Verification items for the finished model (mm, model axes). A direction names the side the tool comes from. Round coordinates to 2 decimals unless told otherwise and drop trailing zeros. Loops run counter-clockwise (first coordinate to the right, second up) from the corner with the lowest first, then second, coordinate; pieces in that order, holes last. Notation, with made-up numbers: (0, -16.5) -> (35, -16.5) arc R19 cw to (35, 16.5) -> close; hole circle Ø7 at (-38, 54). An arc over 180 degrees is marked (long way). Use CSV: the item, a comma, the result in double quotes. Start each with the question number.
```python
from build123d import *

# Parameters (mm, degrees)
SKETCH1_R           = 42.875795621
BOSS_EXTRUDE1_DEPTH = 6
BOSS_EXTRUDE2_DEPTH = 1.5
CUT_EXTRUDE1_REACH  = 62.932
CUT_EXTRUDE2_DEPTH  = 4
CIRPATTERN1_COUNT   = 4
CUT_EXTRUDE3_REACH  = 62.802
SKETCH5_R           = 1.375


with BuildPart() as part:
    # Sketch1 → Boss-Extrude1 (new body)
    with BuildSketch(Plane(origin=(0, 0, 0), x_dir=(1, 0, 0), z_dir=(0, 1, 0))):
        with Locations(Location((0, 0, 0), (0, 0, 270))):
            Circle(SKETCH1_R)
        Polygon((-20.109572639, -34.251708263), (-34.251708263, -20.109572639), (4.639164702, 18.781300326), (18.781300326, 4.639164702), align=None, mode=Mode.SUBTRACT)
    extrude(amount=BOSS_EXTRUDE1_DEPTH)

    # Sketch1<4> → Boss-Extrude2 (add)
    with BuildSketch(Plane(origin=(0, 0, 0), x_dir=(1, 0, 0), z_dir=(0, 1, 0))):
        Polygon((18.781300326, 4.639164702), (4.639164702, 18.781300326), (-0.664136157, 13.477999467), (13.477999467, -0.664136157), align=None)
        Polygon((-14.80627178, -28.948407404), (-28.948407404, -14.80627178), (-34.251708263, -20.109572639), (-20.109572639, -34.251708263), align=None)
    extrude(amount=BOSS_EXTRUDE2_DEPTH)

    # Sketch2 → Cut-Extrude1 (cut, up to next)
    with BuildSketch(Plane(origin=(0, 6, 0), x_dir=(1, 0, 0), z_dir=(0, 1, 0)), mode=Mode.PRIVATE) as cut_extrude1_sk1:
        Polygon((-32.676453, 12.877463126), (-12.877463126, 32.676453), (-8.634822439, 28.433812313), (-28.433812313, 8.634822439), align=None)
    cut_extrude1_tool1 = extrude(cut_extrude1_sk1.sketch, amount=-CUT_EXTRUDE1_REACH, mode=Mode.PRIVATE) & part.part
    add(cut_extrude1_tool1.solids().sort_by_distance((-20.655638, 6, -20.655638))[0], mode=Mode.SUBTRACT)

    # Sketch3 → Cut-Extrude2 (cut)
    with BuildSketch(Plane.XZ):
        with BuildLine():
            Line((-39.625795621, -2.5), (-39.625795621, 2.5))
            ThreePointArc((-39.625795621, 2.5), (-38.875795621, 3.25), (-38.125795621, 2.5))
            Line((-38.125795621, 2.5), (-38.125795621, -2.5))
            ThreePointArc((-38.125795621, -2.5), (-38.875795621, -3.25), (-39.625795621, -2.5))
        make_face()
    cut_extrude2 = extrude(amount=-CUT_EXTRUDE2_DEPTH, mode=Mode.SUBTRACT)

    # CirPattern1: Cut-Extrude2 ×4 about axis
    cirpattern1_axis = Axis((0, 0, 0), (0, 1, 0))
    for i in range(1, CIRPATTERN1_COUNT):
        add(cut_extrude2.rotate(cirpattern1_axis, i * 360 / CIRPATTERN1_COUNT), mode=Mode.SUBTRACT)

    # Sketch5 → Cut-Extrude3 (cut, up to next)
    with BuildSketch(Plane(origin=(0, 1.5, 0), x_dir=(1, 0, 0), z_dir=(0, 1, 0)), mode=Mode.PRIVATE) as cut_extrude3_sk1:
        with Locations(Location((13.301222772, 6.23015496, 0), (0, 0, 270))):
            Circle(SKETCH5_R)
    cut_extrude3_tool1 = extrude(cut_extrude3_sk1.sketch, amount=-CUT_EXTRUDE3_REACH, mode=Mode.PRIVATE) & part.part
    # Sketch5 → Cut-Extrude3 (cut, up to next)
    with BuildSketch(Plane(origin=(0, 1.5, 0), x_dir=(1, 0, 0), z_dir=(0, 1, 0)), mode=Mode.PRIVATE) as cut_extrude3_sk2:
        with Locations(Location((6.23015496, 13.301222772, 0), (0, 0, 270))):
            Circle(SKETCH5_R)
    cut_extrude3_tool2 = extrude(cut_extrude3_sk2.sketch, amount=-CUT_EXTRUDE3_REACH, mode=Mode.PRIVATE) & part.part
    cut_extrude3_1 = cut_extrude3_tool1.solids().sort_by_distance((13.301223, 1.5, -6.230155))[0]
    add(cut_extrude3_1, mode=Mode.SUBTRACT)
    cut_extrude3_2 = cut_extrude3_tool2.solids().sort_by_distance((6.230155, 1.5, -13.301223))[0]
    add(cut_extrude3_2, mode=Mode.SUBTRACT)
    cut_extrude3 = cut_extrude3_1 + cut_extrude3_2  # Cut-Extrude3 as one shape, for the pattern or mirror that repeats it

    # Mirror1: Cut-Extrude3 across plane
    add(cut_extrude3.mirror(Plane(origin=(-7.735203969, 0, 7.735203969), x_dir=(0.7071067811865474, 0, 0.7071067811865478), z_dir=(-0.7071067811865479, 0, 0.7071067811865472))), mode=Mode.SUBTRACT)


solid = part.part
```
Q1. Cross-section at A-A (y = 3). Record the boundary of the cut face in (x, z).
Q2. Tool access check on faces 4 (the face through (-25, 1.5, 24)), 5 (the face through (6.308, 0.74, -6.506)), 6 (the face through (38.126, 2, 0)). Record the directions out of +Z, -Z, +X, -X, +Y, -Y that give a thin tool (end or side, any length) a straight path to the whole face; none if there is none.
Q3. Cross-section at B-B (z = 17). Record the boundary of the cut face in (x, y), and give its area (3 significant figures).
Q4. Cross-section at C-C (x = -17). Record the boundary of the cut face in (y, z).
Q5. Depth check by flat-ended pin: pin 1 Ø4.5 at (x, z) = (13.3, -6.23) entering from +Y; pin 2 Ø2 at (x, z) = (-21.7, 28.77) entering from -Y; pin 3 Ø1 at (x, y) = (23.5, 5) entering from -Z; pin 4 Ø2 at (x, y) = (-15.5, 5) entering from +Z. Enter the tip coordinate at first touch or a pass-through.
Q6. Release check for a two-part mould opening along Z. For faces 1 (the face through (10, 6, 9)), 2 (the face through (-26.089, 2.958, -34.025)), 3 (the face through (-28.951, 0.76, 23.064)) record: +Z half, -Z half, draft (parallel to the pull), parting line (faces both ways), or undercut.
Q7. Cross-section at D-D (z = 33). Record the boundary of the cut face in (x, y).
Q8. Thickness scan on L1, parallel to X at y = 3.5, z = -16; L2, parallel to X at y = 2.75, z = -1; L3, parallel to Z at x = 12.5, y = 0.5. Record the ranges inside material, lowest first. Write a range as from..to.
Answer list:
1,outline,"circle Ø85.75 at (0, 0); hole (-39.63, -2.5) arc R0.75 ccw to (-38.13, -2.5) -> (-38.13, 2.5) arc R0.75 ccw to (-39.63, 2.5) -> close; hole (-34.25, 20.11) -> (4.64, -18.78) -> (18.78, -4.64) -> (-20.11, 34.25) -> close; hole (-32.68, -12.88) -> (-12.88, -32.68) -> (-8.63, -28.43) -> (-28.43, -8.63) -> close; hole (-2.5, -39.63) -> (2.5, -39.63) arc R0.75 ccw to (2.5, -38.13) -> (-2.5, -38.13) arc R0.75 ccw to start; hole (-2.5, 38.13) -> (2.5, 38.13) arc R0.75 ccw to (2.5, 39.63) -> (-2.5, 39.63) arc R0.75 ccw to start; hole (38.13, -2.5) arc R0.75 ccw to (39.63, -2.5) -> (39.63, 2.5) arc R0.75 ccw to (38.13, 2.5) -> close"
2,face 4,"+Y"
2,face 5,"+Y, -Y"
2,face 6,"-Y"
3,outline,"(-39.36, 0) -> (-26.75, 0) -> (-26.75, 1.5) -> (-31.14, 1.5) -> (-31.14, 6) -> (-39.36, 6) -> close; (-2.86, 0) -> (39.36, 0) -> (39.36, 6) -> (-2.86, 6) -> close"
3,area,"309 mm2"
4,outline,"(0, -39.36) -> (6, -39.36) -> (6, -28.55) -> (0, -28.55) -> close; (0, -20.07) -> (6, -20.07) -> (6, 2.86) -> (0, 2.86) -> close; (0, 26.75) -> (1.5, 26.75) -> (1.5, 31.14) -> (6, 31.14) -> (6, 39.36) -> (0, 39.36) -> close"
5,pin 1,"stops at y = 1.5"
5,pin 2,"passes through"
5,pin 3,"stops at z = -36.18"
5,pin 4,"stops at z = 40.35"
6,face 1,"draft"
6,face 2,"parting line"
6,face 3,"undercut"
7,outline,"(-27.37, 0) -> (27.37, 0) -> (27.37, 6) -> (-18.86, 6) -> (-18.86, 1.5) -> (-21.36, 1.5) -> (-21.36, 6) -> (-27.37, 6) -> close"
8,L1,"x = -39.78..-29.55, -21.07..1.86, 7.42..39.78"
8,L2,"x = -42.86..-39.63, -38.13..-13.14, 15.14..38.13, 39.63..42.86"
8,L3,"z = -41.01..-7.35, -5.11..-0.31, 1.64..41.01"
